The listing builds one solid part. Answer for the finished solid, in the listing's coordinates (mm). A direction names the side the tool comes from. Coordinates: 2 decimals unless noted, no trailing zeros. Order: outer loops, then holes, each group sorted by start corner. A loop starts at its lowest first (then second) coordinate and runs counter-clockwise, first axis right, second up. Notation, with made-up numbers: (43, 85.5) - (75, 85.5) arc R25 ccw to (75, 116.5) - close; hole circle Ø5 at (64, 31.5). An arc over 180 degrees is marked (long way). Use one line per item in the form item = value. Start each with the question number.
Item 1: Section B-B, the plane z = 3.75 is taken. Write down the section's boundary in (x, y).
Item 2: The mould has two halves that part along X. Classify faces 1 (the flat face through (19, 0, 6)), 2 (the flat face through (0, -15, 7)), 3 (the cylindrical face through (-17.14, 12.1, 8.41)): released by +X, released by -X, zero draft, split by the parting line, or undercut.
Item 3: Section C-C, the plane y = -7.5 is taken. Write down the section's boundary in (x, z), and give its area (3 significant figures).
Item 4: Consider line 1 along Y through (x, z) = (-10, 7.5); line 2 along X through (y, z) = (-0.5, 5); line 3 along X through (y, z) = (1.5, 4.75). Determine where each line is inside the solid, lowest interval first. Write a range as [from, to].
Item 5: Each of these flat-tipped pins is pushed along its axis until it touches: pin 1 Ø1.6 at (y, z) = (0, 7.5) entering from +X; pin 2 Ø8 at (x, y) = (-12.5, -1) entering from +Z; pin 3 Ø5.5 at (y, z) = (0, 7.5) entering from +X. Where does it stop, or does it pass through?
Item 6: A tool of negligible diameter and unlimited length cuts with its end or side. For faces 4 (the flat face through (0, 0, 2)), 5 (the cylindrical face through (-19, -13, 8)), 6 (the cylindrical face through (18.49, 0.13, 8.49)), from which of +Z, -Z, +X, -X, +Y, -Y can it reach the whole face along a straight path? Write none if from no direction.
Item 7: Section A-A, the plane y = 0 is taken. Write down the section's boundary in (x, z), and give its area (3 significant figures).
Item 8: Section D-D, the plane x = 12.5 is taken. Write down the section's boundary in (y, z).
from build123d import *

# Parameters (mm, degrees)
F0_W           = 40
F0_H           = 30
F1_DEPTH       = 15
F2_T           = -2
F3_R           = 5
F4_R           = 3
F6_D           = 2
F6_DEPTH       = 12
F6_CBORE_D     = 6
F6_CBORE_DEPTH = 1
F6_TIP         = 0.600860619


with BuildPart() as f1:
    # F0 (on Top) → F1 (new body)
    with BuildSketch(Plane.XY):
        Rectangle(F0_W, F0_H)
    extrude(amount=F1_DEPTH)

    # F2
    f2_openings = [f1.faces().sort_by_distance(p)[0] for p in [
        (0, 0, 15),
    ]]
    offset(amount=F2_T, openings=f2_openings)

    # F3
    f3_edges = [f1.edges().sort_by_distance(p)[0] for p in [
        (20, -15, 7.5),
        (20, 15, 7.5),
        (-20, -15, 7.5),
        (-20, 15, 7.5),
    ]]
    fillet(f3_edges, radius=F3_R)

    # F4
    f4_edges = [f1.edges().sort_by_distance(p)[0] for p in [
        (-18, 13, 8.5),
        (-18, -13, 8.5),
        (18, 13, 8.5),
        (18, -13, 8.5),
    ]]
    fillet(f4_edges, radius=F4_R)

    # F6
    with Locations(Plane.YZ.offset(20)):
        with Locations((0, 7.5)):
            CounterBoreHole(F6_D / 2, F6_CBORE_D / 2, F6_CBORE_DEPTH, depth=F6_DEPTH)
            with Locations((0, 0, -(F6_DEPTH + F6_TIP / 2))):  # 118° drill point
                Cone(0, F6_D / 2, F6_TIP, mode=Mode.SUBTRACT)


solid = f1.part
Response:
q1.outline = (-20, -10) arc R5 ccw to (-15, -15) - (15, -15) arc R5 ccw to (20, -10) - (20, 10) arc R5 ccw to (15, 15) - (-15, 15) arc R5 ccw to (-20, 10) - close; hole (-18, -10) arc R3 ccw to (-15, -13) - (15, -13) arc R3 ccw to (18, -10) - (18, 10) arc R3 ccw to (15, 13) - (-15, 13) arc R3 ccw to (-18, 10) - close
q2.face_1 = released by +X
q2.face_2 = zero draft
q2.face_3 = undercut
q3.outline = (-20, 0) - (20, 0) - (20, 15) - (18, 15) - (18, 2) - (-18, 2) - (-18, 15) - (-20, 15) - close
q3.area = 132 mm2
q4.line_1 = [-15, -13], [13, 15]
q4.line_2 = [-20, -18], [18, 19]
q4.line_3 = [-20, -18], [18, 20]
q5.pin_1 = -18
q5.pin_2 = 2
q5.pin_3 = 19
q6.face_4 = +Z
q6.face_5 = +Z, -Z, -X, -Y
q6.face_6 = +X
q7.outline = (-20, 0) - (20, 0) - (20, 4.5) - (19, 4.5) - (19, 6.5) - (18, 6.5) - (18, 2) - (-18, 2) - (-18, 15) - (-20, 15) - close; (18, 8.5) - (19, 8.5) - (19, 10.5) - (20, 10.5) - (20, 15) - (18, 15) - close
q7.area = 124 mm2
q8.outline = (-15, 0) - (15, 0) - (15, 15) - (13, 15) - (13, 2) - (-13, 2) - (-13, 15) - (-15, 15) - close
